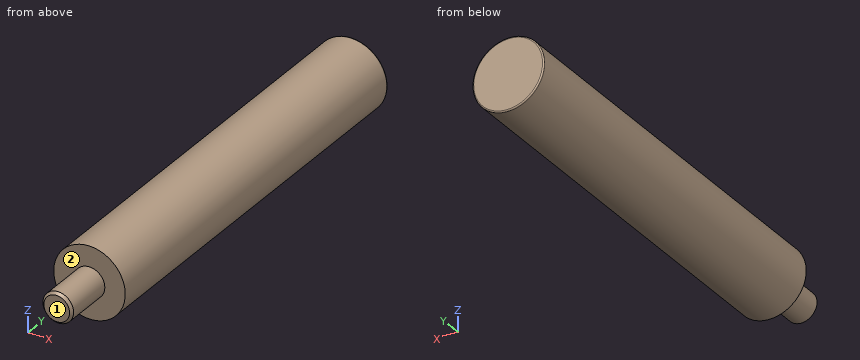
from build123d import *

# Parameters (mm, degrees)
SKETCH1_R           = 14
BOSS_EXTRUDE1_DEPTH = 160
SKETCH2_R           = 10
BOSS_EXTRUDE2_DEPTH = 20
FILLET1_R           = 0.5


# Read off the part's stored shape, not the designer's step: M12 Machine Threads Stud1
with BuildPart() as part:
    # Sketch1 → Boss-Extrude1 (new body)
    with BuildSketch(Plane(origin=(0, 0, 0), x_dir=(1, 0, 0), z_dir=(0, 1, 0))):
        with Locations(Location((0, 0, 0), (0, 0, 270))):
            Circle(SKETCH1_R)
    extrude(amount=BOSS_EXTRUDE1_DEPTH)

    # Sketch2 → Boss-Extrude2 (add)
    with BuildSketch(Plane.XZ):
        with Locations(Location((0, 0, 0), (0, 0, 270))):
            Circle(SKETCH2_R)
    extrude(amount=BOSS_EXTRUDE2_DEPTH)

    # M12 Machine Threads Stud1 outline → M12 Machine Threads Stud1 (revolve, cut)
    with BuildSketch(Plane.XY):
        Polygon((10, 0), (6, 0), (6, -19.036), (5.036, -20), (10, -20), align=None)
    revolve(axis=Axis((0, 0, 0), (0, 1, 0)), mode=Mode.SUBTRACT)

    # Fillet1
    fillet1_edges = [part.edges().sort_by_distance(p)[0] for p in [
        (0, 160, -14),
    ]]
    fillet(fillet1_edges, radius=FILLET1_R)


solid = part.part
Geometry: final body of the model. Coordinates: model frame, mm. Face numbers are marked on the shaded views. A direction names the side the tool comes from. Round coordinates to 2 decimals unless told otherwise and drop trailing zeros. Loops run counter-clockwise (first coordinate to the right, second up) from the corner with the lowest first, then second, coordinate; pieces in that order, holes last.
Q1. Section C-C on y = 5. Return loops of the section in (x, z).
Q2. Material intervals for L1, parallel to Y at x = -5, z = -10.75; L2, parallel to Z at x = -9.25, y = 34.5; L3, parallel to X at y = 89.5, z = -4.75, sorted ascending.
Q3. Access query for the marked faces 1 and 2. Directions: +Z, -Z, +X, -X, +Y, -Y. A direction counts if a zero-diameter tool reaches every point of the face in a straight line with its end or side. Return the directions, or none.
Q4. Section B-B on z = 0. Return loops of the section in (x, y), plus the area to 3 significant figures.
Q5. Pin query (flat end, axial travel): P1, Ø3, axis at y = 108.5, z = 10, coming from the -X side; P2, Ø4, axis at x = -9, z = 6, coming from the -Y side; P3, Ø5, axis at y = 95.5, z = 4, coming from the -X side. Return the tip coordinate at first contact, or that it passes through.
Q6. Section A-A on x = 0. Return loops of the section in (y, z), plus the area to 3 significant figures.
Evaluation:
1. outline: circle Ø28 at (0, 0)
2. L1: y = 0 to 160
2. L2: z = -10.51 to 10.51
2. L3: x = -13.17 to 13.17
3. face 1: +Z, -Z, +X, -X, -Y
3. face 2: -Y
4. outline: (-14, 0) - (-6, 0) - (-6, -19.04) - (-5.04, -20) - (5.04, -20) - (6, -19.04) - (6, 0) - (14, 0) - (14, 159.5) arc R0.5 ccw to (13.5, 160) - (-13.5, 160) arc R0.5 ccw to (-14, 159.5) - close
4. area: 4,720 mm2
5. P1: stops at x = -11.12
5. P2: stops at y = 0
5. P3: stops at x = -13.92
6. outline: (-20, -5.04) - (-19.04, -6) - (0, -6) - (0, -14) - (159.5, -14) arc R0.5 ccw to (160, -13.5) - (160, 13.5) arc R0.5 ccw to (159.5, 14) - (0, 14) - (0, 6) - (-19.04, 6) - (-20, 5.04) - close
6. area: 4,720 mm2
